Part model, mm, in its own coordinate system. Round coordinates to 2 decimals unless told otherwise and drop trailing zeros. Loops run counter-clockwise (first coordinate to the right, second up) from the corner with the lowest first, then second, coordinate; pieces in that order, holes last. Notation, with made-up numbers: (-21.75, 7.25) - (31.25, 7.25) arc R33 ccw to (31.25, 46.25) - close; hole circle Ø6 at (14.25, 61.5). An arc over 180 degrees is marked (long way). Write each question's results on one line, items separated by ' | '. Start each with the question number.
(1) Cut at D-D, the plane y = -5.75. List the corners of the cut face in (x, z), then the cut area to 3 significant figures.
(2) Drill centre lines: L1, parallel to Y at x = 1.75, z = 0; L2, parallel to Z at x = 2, y = 1; L3, parallel to Y at x = 1.2, z = 39.5. Where is each one in solid material? Low to high.
(3) Cut at A-A, the plane y = -1. List the corners of the cut face in (x, z).
(4) Cut at B-B, the plane x = 1.7. List the corners of the cut face in (y, z), then the cut area to 3 significant figures.
(5) Mould opens along Z. For faces 1 (the face through (1, 0, 47)), 2 (the face through (1, -7, 20)), 3 (the face through (1.23, 0.07, 41.5)), 4 (the face through (1.23, 0.07, 1.5)) say: released by +Z, released by -Z, zero draft, split by the parting line, or undercut.
(6) Flat gauge pin, fed straight in: P1, Ø4, axis at y = 0, z = 0, coming from the -X side. Where does the tip first touch, or does it go through?
(7) Cut at C-C, the plane y = -3.25. List the corners of the cut face in (x, z), then the cut area to 3 significant figures.
from build123d import *

# Parameters (mm, degrees)
SKETCH1_R           = 1.5
BOSS_EXTRUDE1_DEPTH = 2.5


with BuildPart() as part:
    # Sketch1 → Boss-Extrude1 (new body)
    with BuildSketch(Plane(origin=(0, 0, 0), x_dir=(0, 0, -1), z_dir=(1, 0, 0))):
        with BuildLine():
            Line((0, -7), (-40, -7))
            ThreePointArc((-40, -7), (-47, 0), (-40, 7))
            Line((-40, 7), (0, 7))
            ThreePointArc((0, 7), (7, 0), (0, -7))
        make_face()
        with Locations((-40, 0)):
            Circle(SKETCH1_R, mode=Mode.SUBTRACT)
        Circle(SKETCH1_R, mode=Mode.SUBTRACT)
    extrude(amount=BOSS_EXTRUDE1_DEPTH)


solid = part.part
A:
1) outline: (0, -3.99) - (2.5, -3.99) - (2.5, 43.99) - (0, 43.99) - close | area: 120 mm2
2) L1: -7 to -1.5, 1.5 to 7 | L2: -6.93 to -1.12, 1.12 to 38.88, 41.12 to 46.93 | L3: -7 to -1.41, 1.41 to 7
3) outline: (0, -6.93) - (2.5, -6.93) - (2.5, -1.12) - (0, -1.12) - close; (0, 1.12) - (2.5, 1.12) - (2.5, 38.88) - (0, 38.88) - close; (0, 41.12) - (2.5, 41.12) - (2.5, 46.93) - (0, 46.93) - close
4) outline: (-7, 0) arc R7 ccw to (7, 0) - (7, 40) arc R7 ccw to (-7, 40) - close; hole circle Ø3 at (0, 0); hole circle Ø3 at (0, 40) | area: 700 mm2
5) face 1: released by +Z | face 2: zero draft | face 3: undercut | face 4: undercut
6) P1: x = 0
7) outline: (0, -6.2) - (2.5, -6.2) - (2.5, 46.2) - (0, 46.2) - close | area: 131 mm2
